Verification items for this drawing (mm, ordinates from the low corner). Round coordinates to 2 decimals unless told otherwise and drop trailing zeros. Write each loop counter-clockwise with the first axis right and the second up, starting at its lowest first coordinate (ties: lowest second). Pieces come first, ordered by that corner, then holes. Notation, with made-up numbers: M 13.5,80.5 L 32.5,80.5 A16 cw 32.5,90.5 Z; hole C 20.5,35 d2. An arc over 180 degrees is marked long. One line per question, with ' | ' between items. Start each with the question number.
Q1. Thickness scan on line 1 along X through (y, z) = (0.3, 59); line 2 along X through (y, z) = (2.15, 49). Record the ranges inside material, lowest first. Write a range as from..to.
Q2. Cross-section at A-A (y = 0.95). Record the boundary of the cut face in (x, z).
Q3. Cross-section at C-C (x = 36). Record the boundary of the cut face in (y, z).
Q4. Cross-section at B-B (z = 46). Record the boundary of the cut face in (x, y).
Q5. Cross-section at D-D (x = 59). Record the boundary of the cut face in (y, z), then the cut area to 3 significant figures.
Q6. Gauge pin test, flat end, axial feed: pin 1 (1.1 mm diameter, centred on x = 15, z = 59, fed in from -Y). Record the tip position at first contact, or that the pin passes through.
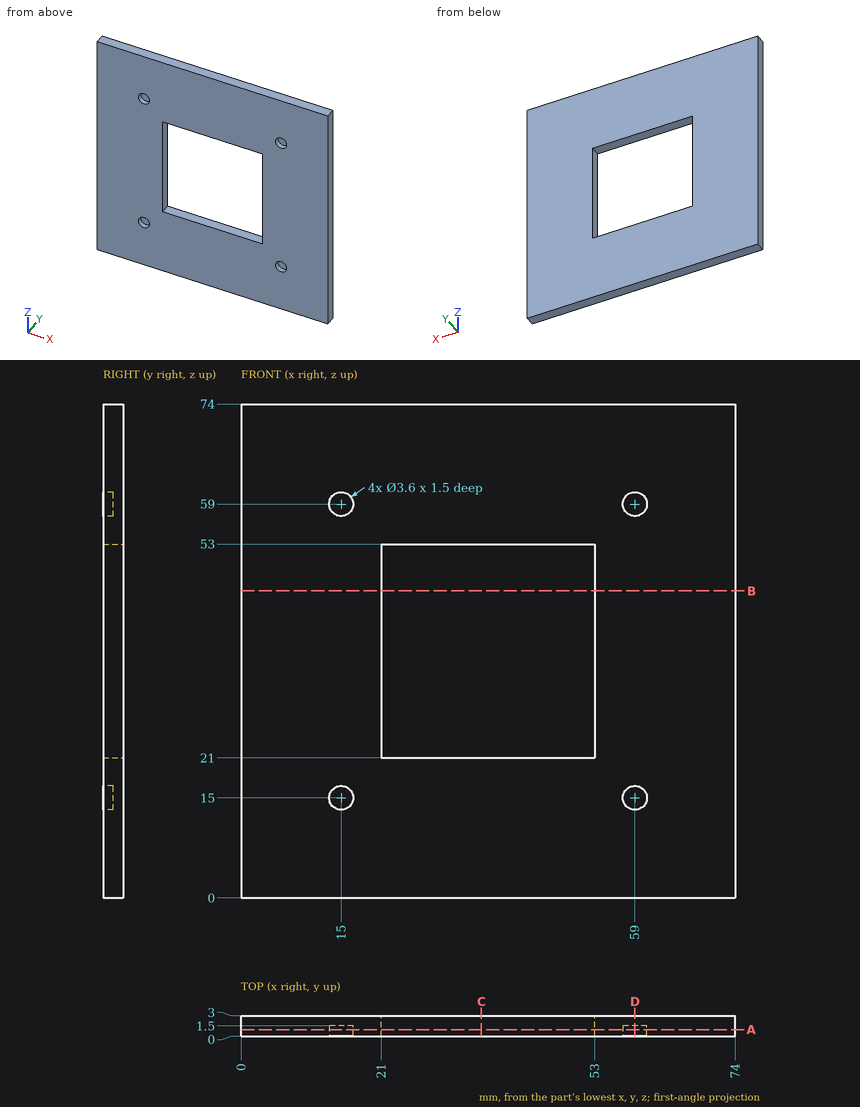
Determined:
1) line 1: x = 0..13.2, 16.8..57.2, 60.8..74 | line 2: x = 0..21, 53..74
2) outline: M 0,0 L 74,0 L 74,74 L 0,74 Z; hole C 15,15 d3.6; hole C 15,59 d3.6; hole M 21,21 L 53,21 L 53,53 L 21,53 Z; hole C 59,15 d3.6; hole C 59,59 d3.6
3) outline: M 0,0 L 3,0 L 3,21 L 0,21 Z; M 0,53 L 3,53 L 3,74 L 0,74 Z
4) outline: M 0,0 L 21,0 L 21,3 L 0,3 Z; M 53,0 L 74,0 L 74,3 L 53,3 Z
5) outline: M 0,0 L 3,0 L 3,74 L 0,74 L 0,60.8 L 1.5,60.8 L 1.5,57.2 L 0,57.2 L 0,16.8 L 1.5,16.8 L 1.5,13.2 L 0,13.2 Z | area: 211 mm²
6) pin 1: stops at y = 1.5
